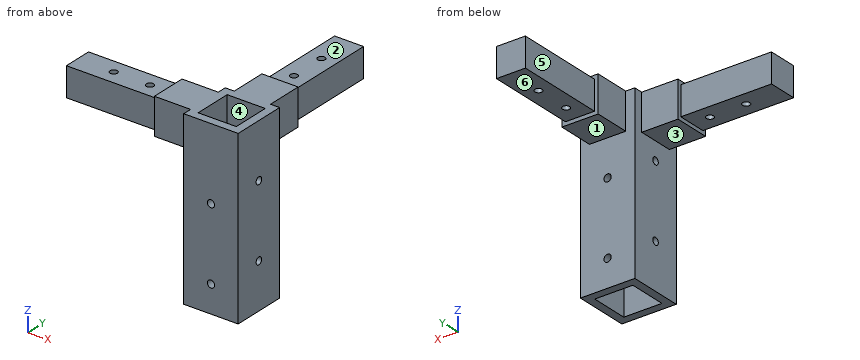
```python
from build123d import *

# Parameters (mm, degrees)
SKETCH1_W           = 100
SKETCH1_H           = 100
BOSS_EXTRUDE1_DEPTH = 100
CUT_EXTRUDE16_DEPTH = 70
SKETCH8_W           = 70
SKETCH8_H           = 70
CUT_EXTRUDE17_DEPTH = 30
SKETCH9_W           = 21
SKETCH9_H           = 21
CUT_EXTRUDE20_DEPTH = 100
SKETCH10_W          = 30
SKETCH10_H          = 30
SKETCH10_W_2        = 16
SKETCH10_H_2        = 16
CUT_EXTRUDE21_DEPTH = 50
SKETCH11_W          = 30
SKETCH11_H          = 30
SKETCH11_W_2        = 20
SKETCH11_H_2        = 20
CUT_EXTRUDE22_DEPTH = 20
SKETCH12_W          = 30
SKETCH12_H          = 30
SKETCH12_W_2        = 20
SKETCH12_H_2        = 20
CUT_EXTRUDE23_DEPTH = 70
SKETCH13_W          = 20
SKETCH13_H          = 20
SKETCH13_W_2        = 16
SKETCH13_H_2        = 16
CUT_EXTRUDE24_DEPTH = 50
SKETCH15_R          = 2
CUT_EXTRUDE25_DEPTH = 30
SKETCH16_R          = 2
CUT_EXTRUDE26_DEPTH = 30
SKETCH17_R          = 2
CUT_EXTRUDE27_DEPTH = 16
SKETCH18_R          = 2
CUT_EXTRUDE29_DEPTH = 16
SKETCH19_W          = 30
SKETCH19_H          = 30
CUT_EXTRUDE30_DEPTH = 5


with BuildPart() as part:
    # Sketch1 → Boss-Extrude1 (new body)
    with BuildSketch(Plane.XY):
        Rectangle(SKETCH1_W, SKETCH1_H)
    extrude(amount=-BOSS_EXTRUDE1_DEPTH)

    # Sketch5 → Cut-Extrude16 (cut)
    with BuildSketch(Plane(origin=(0, 0, -100), x_dir=(-1, 0, 0), z_dir=(0, 0, -1))):
        Polygon((50, -50), (50, 50), (-50, 50), (-50, -20), (-20, -20), (-20, -50), align=None)
    extrude(amount=-CUT_EXTRUDE16_DEPTH, mode=Mode.SUBTRACT)

    # Sketch8 → Cut-Extrude17 (cut)
    with BuildSketch(Plane(origin=(0, 0, -30), x_dir=(-1, 0, 0), z_dir=(0, 0, -1))):
        with Locations((15, 15)):
            Rectangle(SKETCH8_W, SKETCH8_H)
    extrude(amount=-CUT_EXTRUDE17_DEPTH, mode=Mode.SUBTRACT)

    # Sketch9 → Cut-Extrude20 (cut)
    with BuildSketch(Plane(origin=(0, 0, -100), x_dir=(-1, 0, 0), z_dir=(0, 0, -1))):
        with Locations((-35, -35)):
            Rectangle(SKETCH9_W, SKETCH9_H)
    extrude(amount=-CUT_EXTRUDE20_DEPTH, mode=Mode.SUBTRACT)

    # Sketch10 → Cut-Extrude21 (cut)
    with BuildSketch(Plane.ZY.offset(50)):
        with Locations((-15, -35)):
            Rectangle(SKETCH10_W, SKETCH10_H)
        with Locations((-15, -35)):
            Rectangle(SKETCH10_W_2, SKETCH10_H_2, mode=Mode.SUBTRACT)
    extrude(amount=-CUT_EXTRUDE21_DEPTH, mode=Mode.SUBTRACT)

    # Sketch11 → Cut-Extrude22 (cut)
    with BuildSketch(Plane.ZY):
        with Locations((-15, -35)):
            Rectangle(SKETCH11_W, SKETCH11_H)
        with Locations((-15, -35)):
            Rectangle(SKETCH11_W_2, SKETCH11_H_2, mode=Mode.SUBTRACT)
    extrude(amount=-CUT_EXTRUDE22_DEPTH, mode=Mode.SUBTRACT)

    # Sketch12 → Cut-Extrude23 (cut)
    with BuildSketch(Plane(origin=(0, 50, 0), x_dir=(1, 0, 0), z_dir=(0, 1, 0))):
        with Locations((35, 15)):
            Rectangle(SKETCH12_W, SKETCH12_H)
        with Locations((35, 15)):
            Rectangle(SKETCH12_W_2, SKETCH12_H_2, mode=Mode.SUBTRACT)
    extrude(amount=-CUT_EXTRUDE23_DEPTH, mode=Mode.SUBTRACT)

    # Sketch13 → Cut-Extrude24 (cut)
    with BuildSketch(Plane(origin=(0, 50, 0), x_dir=(1, 0, 0), z_dir=(0, 1, 0))):
        with Locations((35, 15)):
            Rectangle(SKETCH13_W, SKETCH13_H)
        with Locations((35, 15)):
            Rectangle(SKETCH13_W_2, SKETCH13_H_2, mode=Mode.SUBTRACT)
    extrude(amount=-CUT_EXTRUDE24_DEPTH, mode=Mode.SUBTRACT)

    # Sketch15 → Cut-Extrude25 (cut)
    with BuildSketch(Plane(origin=(0, -20, 0), x_dir=(1, 0, 0), z_dir=(0, 1, 0))):
        with Locations(Location((35, 85, 0), (0, 0, 270))):
            Circle(SKETCH15_R)
        with Locations(Location((35, 45, 0), (0, 0, 270))):
            Circle(SKETCH15_R)
    extrude(amount=-CUT_EXTRUDE25_DEPTH, mode=Mode.SUBTRACT)

    # Sketch16 → Cut-Extrude26 (cut)
    with BuildSketch(Plane(origin=(50, 0, 0), x_dir=(0, 0, -1), z_dir=(1, 0, 0))):
        with Locations((75, -35)):
            Circle(SKETCH16_R)
        with Locations((35, -35)):
            Circle(SKETCH16_R)
    extrude(amount=-CUT_EXTRUDE26_DEPTH, mode=Mode.SUBTRACT)

    # Sketch17 → Cut-Extrude27 (cut)
    with BuildSketch(Plane(origin=(0, 0, -23), x_dir=(-1, 0, 0), z_dir=(0, 0, -1))):
        with Locations((-35, 30)):
            Circle(SKETCH17_R)
        with Locations((-35, 10)):
            Circle(SKETCH17_R)
    extrude(amount=-CUT_EXTRUDE27_DEPTH, mode=Mode.SUBTRACT)

    # Sketch18 → Cut-Extrude29 (cut)
    with BuildSketch(Plane(origin=(0, 0, -23), x_dir=(-1, 0, 0), z_dir=(0, 0, -1))):
        with Locations((30, -35)):
            Circle(SKETCH18_R)
        with Locations((10, -35)):
            Circle(SKETCH18_R)
    extrude(amount=-CUT_EXTRUDE29_DEPTH, mode=Mode.SUBTRACT)

    # Sketch19 → Cut-Extrude30 (cut)
    with BuildSketch(Plane.XY):
        with Locations((35, -35)):
            Rectangle(SKETCH19_W, SKETCH19_H)
    extrude(amount=-CUT_EXTRUDE30_DEPTH, mode=Mode.SUBTRACT)


solid = part.part
```
Can you work these out from the model? Positions are in its coordinate system, mm. Face numbers are marked on the shaded views. A direction names the side the tool comes from. Round coordinates to 2 decimals unless told otherwise and drop trailing zeros. Loops run counter-clockwise (first coordinate to the right, second up) from the corner with the lowest first, then second, coordinate; pieces in that order, holes last. Notation, with made-up numbers: (35.5, 16) -> (78.5, 16) arc R18 cw to (78.5, 23) -> close; hole circle Ø3 at (71, 68.25). An arc over 180 degrees is marked (long way). One line per item, written item: value. Start each with the question number.
1. For pin 1 (10 mm diameter, centred on x = -12.5, y = -39.5, fed in from -Z); pin 2 (6 mm diameter, centred on y = -10, z = -11, fed in from +X); pin 3 (10 mm diameter, centred on x = -33, y = -29, fed in from +Z); pin 4 (2.5 mm diameter, centred on x = 35, y = 10, fed in from -Z), each with a flat end and sliding along its axis, tell me the tip position at first contact or that it passes through.
2. If I drill on probe 1 along Y at (x, z) = (35, -12.75); probe 2 along Y at (x, z) = (45, -58.5); probe 3 along X at (y, z) = (-49, -45), over which ranges is the centre line in solid material (lowest first)?
3. If we section it at D-D, the plane x = 35: Give the number of separate pieces and of enclosed holes in the cut face, then the cut area to 4 significant figures.
4. If we section it at C-C, the plane z = -30.5: Write out the boundary of the cut face in (x, y).
5. For the marked faces 1, 2 and 3, which set-ups out of +Z, -Z, +X, -X, +Y, -Y let a thin tool reach every point of the face, with its end or its side?
6. If we section it at A-A, the plane z = -75: Write out the boundary of the cut face in (x, y), then the cut area to 3 significant figures.
7. If we mould it in two halves opening along X, with no side actions, what happens to the marked faces 4, 5 and 6? For each: pulls with the +X half, pulls with the -X half, needs draft (parallel to the pull), parting line crosses it, or undercut.
8. If we section it at B-B, the plane y = 10: Write out the boundary of the cut face in (x, z), then the cut area to 3 significant figures.
Calculated:
1. pin 1: stops at z = -23
1. pin 2: stops at x = 45
1. pin 3: stops at z = -7
1. pin 4: passes through
2. probe 1: y = -50 to -45.5, -24.5 to 8, 12 to 28, 32 to 50
2. probe 2: y = -50 to -45.5, -24.5 to -20
2. probe 3: x = 20 to 33, 37 to 50
3. separate pieces: 8
3. enclosed holes: 0
3. area: 1,855 mm²
4. outline: (20, -50) -> (50, -50) -> (50, -20) -> (20, -20) -> close; hole (24.5, -45.5) -> (45.5, -45.5) -> (45.5, -24.5) -> (24.5, -24.5) -> close
5. face 1: -Z, +X, -X, +Y
5. face 2: +Z, +X, -X, +Y
5. face 3: -Z, -X, +Y, -Y
6. outline: (20, -50) -> (50, -50) -> (50, -37) -> (45.5, -37) -> (45.5, -45.5) -> (24.5, -45.5) -> (24.5, -37) -> (20, -37) -> close; (20, -33) -> (24.5, -33) -> (24.5, -24.5) -> (45.5, -24.5) -> (45.5, -33) -> (50, -33) -> (50, -20) -> (20, -20) -> close
6. area: 423 mm²
7. face 4: undercut
7. face 5: pulls with the -X half
7. face 6: needs draft
8. outline: (27, -23) -> (33, -23) -> (33, -7) -> (27, -7) -> close; (37, -23) -> (43, -23) -> (43, -7) -> (37, -7) -> close
8. area: 192 mm²
